Read the model definition and answer for the solid it produces. Units are mm, in the model's axes. A direction names the side the tool comes from. Coordinates: 2 decimals unless noted, no trailing zeros. Write each loop counter-clockwise with the first axis right and the second up, starting at its lowest first coordinate (ties: lowest second). Pieces come first, ordered by that corner, then holes. Notation, with made-up numbers: (47, -34) -> (83, -34) arc R27 cw to (83, 2) -> close; hole circle Ø4 at (58, 17.25). An arc over 180 degrees is marked (long way). Answer as a JSON object with one key per item and string values. Group by question number.
(1) Find section A-A (z = 14). Give the vertices of the cut face in (x, y).
(2) Which of the six approach directions +Z, -Z, +X, -X, +Y, -Y give full straight-line access (tool end or side, diameter ignored) to faces 1 (the face through (-45.026, 1, 6)), 2 (the face through (-59, 3, 6))?
(3) Find section C-C (x = -59). Give the vertices of the cut face in (y, z), then the cut area to 3 significant figures.
(4) Straight lines are drawn through the part: L1, parallel to X at y = 17.25, z = -3.75; L2, parallel to Y at x = -59.75, z = 3.75. For each, find the intervals that lie inside material, in ascending order.
(5) Find section B-B (y = 9.5). Give the vertices of the cut face in (x, z), then the cut area to 3 significant figures.
(6) Flat-ended cylindrical pins translate along their axes: P1, Ø13.5, axis at x = -62.5, z = 8.5, coming from the +Y side; P2, Ø3, axis at x = -50.5, z = 3.5, coming from the -Y side; P3, Ø2, axis at y = 13, z = 5.5, coming from the +X side. Find the tip coordinate at first contact, or state that the pin passes through.
from build123d import *

# Parameters (mm, degrees)
SKETCH1_W           = 30
SKETCH1_H           = 30
BOSS_EXTRUDE1_DEPTH = 30
SHELL1_T            = -3


with BuildPart() as part:
    # Sketch1 → Boss-Extrude1 (new body)
    with BuildSketch(Plane(origin=(0, 0, 0), x_dir=(1, 0, 0), z_dir=(0, 1, 0))):
        with Locations((-60.026365989, -5.886774035)):
            Rectangle(SKETCH1_W, SKETCH1_H)
    extrude(amount=BOSS_EXTRUDE1_DEPTH)

    # Shell1
    shell1_openings = [part.faces().sort_by_distance(p)[0] for p in [
        (-60.026365989, 30, 5.886774035),
        (-60.026365989, 15, -9.113225965),
        (-45.026365989, 15, 5.886774035),
        (-60.026365989, 15, 20.886774035),
    ]]
    offset(amount=SHELL1_T, openings=shell1_openings, kind=Kind.INTERSECTION)


solid = part.part
Results below:
{
 "1": {"outline": "(-75.03, 0) -> (-45.03, 0) -> (-45.03, 3) -> (-72.03, 3) -> (-72.03, 30) -> (-75.03, 30) -> close"},
 "2": {"face 1": "+Z, -Z, +X, +Y, -Y", "face 2": "+Z, -Z, +X, +Y"},
 "3": {"outline": "(0, -9.11) -> (3, -9.11) -> (3, 20.89) -> (0, 20.89) -> close", "area": "90.0 mm2"},
 "4": {"L1": "x = -75.03 to -72.03", "L2": "y = 0 to 3"},
 "5": {"outline": "(-75.03, -9.11) -> (-72.03, -9.11) -> (-72.03, 20.89) -> (-75.03, 20.89) -> close", "area": "90.0 mm2"},
 "6": {"P1": "stops at y = 3", "P2": "stops at y = 0", "P3": "stops at x = -72.03"}
}
